```python
from build123d import *

# Parameters (mm, degrees)
F0_R      = 10
F0_R_2    = 2.1
F1_DEPTH  = 7
F2_R      = 9
F3_DEPTH  = 5
F5_DEPTH  = 7
F6_W      = 8.5
F6_H      = 2
F7_DEPTH  = 12.8
F8_W      = 6.5
F8_H      = 5
F9_DEPTH  = 15
F10_W     = 1
F10_H     = 5
F11_DEPTH = 0.5
F12_W     = 1
F12_H     = 5
F13_DEPTH = 0.5
F14_SIZE  = 0.49999
F15_SIZE  = 1


# Not quite as in the source:
# - a fillet or chamfer is up to 0.001 mm smaller than in the source, because OpenCascade refuses the exact size


with BuildPart() as f1:
    # F0 (on Top) → F1 (new body)
    with BuildSketch(Plane.XY):
        Circle(F0_R)
        Circle(F0_R_2, mode=Mode.SUBTRACT)
    extrude(amount=F1_DEPTH)

    # F2 (on face) → F3 (cut)
    with BuildSketch(Plane.XY.offset(7)):
        Circle(F2_R)
    extrude(amount=-F3_DEPTH, mode=Mode.SUBTRACT)

    # F4 (on face) → F5 (join)
    with BuildSketch(Plane.XY.offset(7)):
        with BuildLine():
            Line((-10, 16), (-10, 0))
            ThreePointArc((-10, 0), (-9.7467943448, 2.2360679775), (-9, 4.3588989435))
            Line((-9, 4.3588989435), (-9, 16))
            Line((-9, 16), (-10, 16))
        make_face()
        with BuildLine():
            ThreePointArc((-2.5, 9.6824583655), (-2.0026095485, 9.7974259373), (-1.5, 9.8868599666))
            Line((-1.5, 9.8868599666), (-1.5, 16))
            Line((-1.5, 16), (-2.5, 16))
            Line((-2.5, 16), (-2.5, 9.6824583655))
        make_face()
    extrude(amount=-F5_DEPTH)

    # F6 (on face) → F7 (join)
    with BuildSketch(Plane(origin=(0, 16, 0), x_dir=(-1, 0, 0), z_dir=(0, 1, 0))):
        with Locations((5.75, 1)):
            Rectangle(F6_W, F6_H)
    extrude(amount=-F7_DEPTH)

    # F8 (on face) → F9 (cut)
    with BuildSketch(Plane(origin=(0, 16, 0), x_dir=(-1, 0, 0), z_dir=(0, 1, 0))):
        with Locations((5.75, 4.5)):
            Rectangle(F8_W, F8_H)
    extrude(amount=-F9_DEPTH, mode=Mode.SUBTRACT)

    # F10 (on face) → F11 (join)
    with BuildSketch(Plane.YZ.offset(-9)):
        with Locations((1.5, 4.5)):
            Rectangle(F10_W, F10_H)
        with Locations((15.5, 4.5)):
            Rectangle(F10_W, F10_H)
    extrude(amount=F11_DEPTH)

    # F12 (on face) → F13 (join)
    with BuildSketch(Plane(origin=(-2.5, 0, 0), x_dir=(0, -1, 0), z_dir=(-1, 0, 0))):
        with Locations((-15.5, 4.5)):
            Rectangle(F12_W, F12_H)
    extrude(amount=F13_DEPTH)

    # F14 (size 0.5 in the source; OpenCascade refuses exactly that, so slightly less here)
    f14_edges = [f1.edges().sort_by_distance(p)[0] for p in [
        (-8.5, 1.5, 7),
        (-8.5, 15.5, 7),
        (-3, 15.5, 7),
    ]]
    chamfer(f14_edges, length=F14_SIZE)

    # F15
    f15_edges = [f1.edges().sort_by_distance(p)[0] for p in [
        (7.582875, -6.519202, 0),
        (-1.5, 12.94343, 0),
        (-10, 8, 0),
    ]]
    chamfer(f15_edges, length=F15_SIZE)


solid = f1.part
```
CAD build for the part. Positions are in the model's coordinates, mm. A direction names the side the tool comes from. Round coordinates to 2 decimals unless told otherwise and drop trailing zeros. Order: outer loops, then holes, each group sorted by start corner. A loop starts at its lowest first (then second) coordinate and runs counter-clockwise, first axis right, second up.
Item 1: Mould opens along X. For faces 1 (the face through (-2, 9, 7)), 2 (the face through (-9.5, 8.1, 0.5)), 3 (the face through (2.003, 0.631, 0.986)) say: pulls with the +X half, pulls with the -X half, needs draft (parallel to the pull), parting line crosses it, or undercut.
Item 2: Probe line 1 along X through (y, z) = (10.5, 3.5); line 2 along Y through (x, z) = (0, 3.8); line 3 along Y through (x, z) = (0, 1.5). List the from-to ranges inside material, lowest first.
Item 3: Tool access for faces 4 (the face through (-8.5, 1.5, 4.3)), 5 (the face through (-10, 8, 4)), 6 (the face through (6.67, -6.04, 4.54)): list every direction of +Z, -Z, +X, -X, +Y, -Y with a clear straight run to the whole face (end or side of a thin tool).
Item 4: Saw through at C-C on y = 12.5. Write the cut outline in (x, z), then the cut area to 3 significant figures.
Item 5: Saw through at A-A on x = 0. Write the cut outline in (y, z), then the cut area to 3 significant figures.
Item 6: Pin check, flat tips, straight feed: pin 1 (2.5 mm diameter, centred on y = 11.5, z = 4.5, fed in from +X); pin 2 (2 mm diameter, centred on x = 5.5, z = 4.5, fed in from +Y); pin 3 (4 mm diameter, centred on x = -1, y = -4, fed in from +Z); pin 4 (2.5 mm diameter, centred on x = 0, y = 0, fed in from +Z). Stop position of each tip, or through.
Item 7: Saw through at B-B on z = 4.25. Write the cut outline in (x, y), then the cut area to 3 significant figures.
Item 8: Saw through at D-D on z = 0.5. Write the cut outline in (x, y), then the cut area to 3 significant figures.
Reported:
1. face 1: needs draft
1. face 2: pulls with the -X half
1. face 3: undercut
2. line 1: x = -10 to -9, -2.5 to -1.5
2. line 2: y = -10 to -9, 9 to 10
2. line 3: y = -10 to -2.1, 2.1 to 10
3. face 4: +Z, +Y
3. face 5: +Z, -Z, -X, +Y, -Y
3. face 6: +Z
4. outline: (-10, 1) - (-9, 0) - (-2.5, 0) - (-1.5, 1) - (-1.5, 7) - (-2.5, 7) - (-2.5, 2) - (-9, 2) - (-9, 7) - (-10, 7) - close
4. area: 26.0 mm2
5. outline: (-10, 1) - (-9, 0) - (-2.1, 0) - (-2.1, 2) - (-9, 2) - (-9, 7) - (-10, 7) - close; (2.1, 0) - (9, 0) - (10, 1) - (10, 7) - (9, 7) - (9, 2) - (2.1, 2) - close
5. area: 40.6 mm2
6. pin 1: stops at x = -1.5
6. pin 2: stops at y = 8.93
6. pin 3: stops at z = 2
6. pin 4: passes through
7. outline: (-10, 0) arc R10 ccw (long way) to (-1.5, 9.89) - (-1.5, 16) - (-3, 16) - (-3, 15) - (-2.5, 15) - (-2.5, 8.65) arc R9 cw (long way) to (-8.94, 1) - (-8.5, 1) - (-8.5, 2) - (-9, 2) - (-9, 15) - (-8.5, 15) - (-8.5, 16) - (-10, 16) - close
7. area: 71.0 mm2
8. outline: (-9.5, 0) arc R9.5 ccw (long way) to (-2, 9.29) - (-2, 16) - (-9.5, 16) - close; hole circle Ø4.2 at (0, 0)
8. area: 338 mm2
